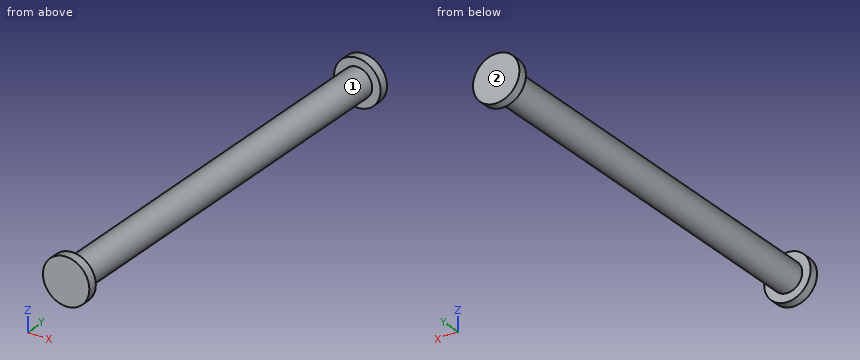
Autodesk Inventor part; units mm, degrees
ref_plane "YZ Plane" through (0, 0, 0) normal (1, 0, 0) x (0, 1, 0)
ref_plane "XZ Plane" through (0, 0, 0) normal (0, 1, 0) x (-1, 0, 0)
ref_plane "XY Plane" through (0, 0, 0) normal (0, 0, 1) x (1, 0, 0)
sketch "Boceto1" plane through (0, 0, 0) normal (0, 1, 0) x (-1, 0, 0)
  circle A0 centre (0, 0) radius 4.8
  circle A1 centre (0, 0) radius 2.8
  dimension "d0" = 9.6
  dimension "d1" = 2
extrude "Extrusión1" add sketch "Boceto1" along normal blind 132
sketch "Boceto2" plane through (0, 132, 0) normal (0, 1, 0) x (1, 0, 0)
  circle A0 centre (0, 0) radius 7.5
  dimension "d4" = 15
extrude "Extrusión2" add sketch "Boceto2" along normal blind 3
sketch "Boceto3" plane through (0, 0, 0) normal (0, -1, 0) x (1, 0, 0)
  circle A0 centre (0, 0) radius 7.5
  dimension "d7" = 15
extrude "Extrusión3" add sketch "Boceto3" along normal blind 3
properties part number "Asiento - Manija" material "Aluminio 6061"
Work out the finished part from the listing and answer in its coordinate system (mm). Face numbers are marked on the shaded views. A direction names the side the tool comes from. Round coordinates to 2 decimals unless told otherwise and drop trailing zeros. Write each loop counter-clockwise with the first axis right and the second up, starting at its lowest first coordinate (ties: lowest second). Pieces come first, ordered by that corner, then holes.
1) Given pin 1 Ø6 at (y, z) = (105, -5.5) entering from +X; pin 2 Ø3 at (x, y) = (5, 109) entering from -Z; pin 3 Ø1 at (x, y) = (4.5, 77.5) entering from -Z, each flat-ended and moving along its own axis, determine where each tip first touches the part or whether it passes through.
2) A cutting plane is placed at B-B (z = 6.25). Give the vertices of the cut face in (x, y).
3) A cutting plane is placed at C-C (z = 0). Give the vertices of the cut face in (x, y).
4) A cutting plane is placed at D-D (y = 97.5). Give the vertices of the cut face in (x, z), plus the area to 3 significant figures.
5) Straight lines are drawn through the part: line 1 (Z direction, x = 0, y = 41.5); line 2 (Y direction, x = -5.5, z = -1); line 3 (X direction, y = 86.5, z = 0.25). For each, find the intervals that lie inside material, in ascending order.
6) A tool of negligible diameter and unlimited length cuts with its end or side. For the marked faces 1 and 2, from which of +Z, -Z, +X, -X, +Y, -Y can it reach the whole face along a straight path? Write none if from no direction.
7) A cutting plane is placed at A-A (x = 0). Give the vertices of the cut face in (y, z).
Completed:
1. pin 1: stops at x = 4.1
1. pin 2: stops at z = -3.28
1. pin 3: stops at z = -2.65
2. outline: (-4.15, -3) - (4.15, -3) - (4.15, 0) - (-4.15, 0) - close; (-4.15, 132) - (4.15, 132) - (4.15, 135) - (-4.15, 135) - close
3. outline: (-7.5, -3) - (7.5, -3) - (7.5, 0) - (4.8, 0) - (4.8, 132) - (7.5, 132) - (7.5, 135) - (-7.5, 135) - (-7.5, 132) - (-4.8, 132) - (-4.8, 0) - (-7.5, 0) - close; hole (-2.8, 0) - (2.8, 0) - (2.8, 132) - (-2.8, 132) - close
4. outline: circle Ø9.6 at (0, 0); hole circle Ø5.6 at (0, 0)
4. area: 47.8 mm2
5. line 1: z = -4.8 to -2.8, 2.8 to 4.8
5. line 2: y = -3 to 0, 132 to 135
5. line 3: x = -4.79 to -2.79, 2.79 to 4.79
6. face 1: none
6. face 2: +Z, -Z, +X, -X, +Y
7. outline: (-3, -7.5) - (0, -7.5) - (0, -4.8) - (132, -4.8) - (132, -7.5) - (135, -7.5) - (135, 7.5) - (132, 7.5) - (132, 4.8) - (0, 4.8) - (0, 7.5) - (-3, 7.5) - close; hole (0, -2.8) - (132, -2.8) - (132, 2.8) - (0, 2.8) - close
